Could you check a few things on this model? Use its own coordinates, in mm. Round coordinates to 2 decimals unless told otherwise and drop trailing zeros. Loops run counter-clockwise (first coordinate to the right, second up) from the corner with the lowest first, then second, coordinate; pieces in that order, holes last. Notation, with made-up numbers: (41, 27) - (57, 27) arc R31 cw to (57, 56) - close; hole circle Ø2 at (-15, 88.5). An arc over 180 degrees is marked (long way). Use one line per item in the form item = value.
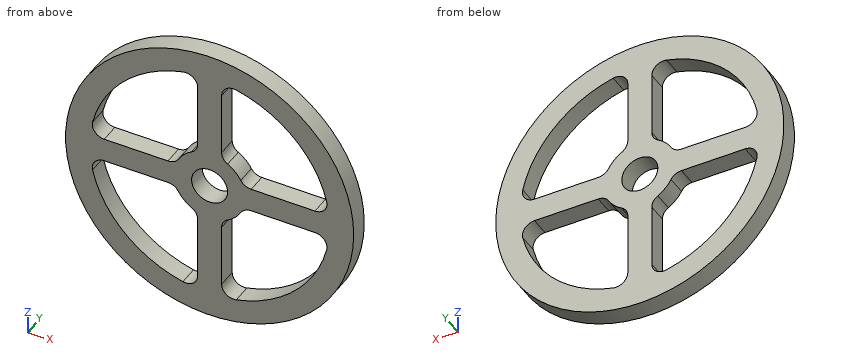
```python
from build123d import *

# Parameters (mm, degrees)
SKETCH1_R           = 120
SKETCH1_R_2         = 15
BOSS_EXTRUDE1_DEPTH = 16


with BuildPart() as part:
    # Sketch1 → Boss-Extrude1 (new body)
    with BuildSketch(Plane(origin=(0, 0, 0), x_dir=(1, 0, 0), z_dir=(0, 1, 0))):
        Circle(SKETCH1_R)
        Circle(SKETCH1_R_2, mode=Mode.SUBTRACT)
        with BuildLine():
            Line((34.641016151, 10), (87.749643874, 10))
            ThreePointArc((87.749643874, 10), (95.567003474, 13.763904355), (97.499604304, 22.222222222))
            ThreePointArc((97.499604304, 22.222222222), (70.710678119, 70.710678119), (22.222222222, 97.499604304))
            ThreePointArc((22.222222222, 97.499604304), (13.763904355, 95.567003474), (10, 87.749643874))
            Line((10, 87.749643874), (10, 34.641016151))
            ThreePointArc((10, 34.641016151), (11.339745962, 29.641016151), (15, 25.980762114))
            ThreePointArc((15, 25.980762114), (21.213203436, 21.213203436), (25.980762114, 15))
            ThreePointArc((25.980762114, 15), (29.641016151, 11.339745962), (34.641016151, 10))
        make_face(mode=Mode.SUBTRACT)
        with BuildLine():
            Line((-10, 34.641016151), (-10, 87.749643874))
            ThreePointArc((-10, 87.749643874), (-13.763904355, 95.567003474), (-22.222222222, 97.499604304))
            ThreePointArc((-22.222222222, 97.499604304), (-70.710678119, 70.710678119), (-97.499604304, 22.222222222))
            ThreePointArc((-97.499604304, 22.222222222), (-95.567003474, 13.763904355), (-87.749643874, 10))
            Line((-87.749643874, 10), (-34.641016151, 10))
            ThreePointArc((-34.641016151, 10), (-29.641016151, 11.339745962), (-25.980762114, 15))
            ThreePointArc((-25.980762114, 15), (-21.213203436, 21.213203436), (-15, 25.980762114))
            ThreePointArc((-15, 25.980762114), (-11.339745962, 29.641016151), (-10, 34.641016151))
        make_face(mode=Mode.SUBTRACT)
        with BuildLine():
            Line((34.641016151, -10), (87.749643874, -10))
            ThreePointArc((87.749643874, -10), (95.567003474, -13.763904355), (97.499604304, -22.222222222))
            ThreePointArc((97.499604304, -22.222222222), (70.710678119, -70.710678119), (22.222222222, -97.499604304))
            ThreePointArc((22.222222222, -97.499604304), (13.763904355, -95.567003474), (10, -87.749643874))
            Line((10, -87.749643874), (10, -34.641016151))
            ThreePointArc((10, -34.641016151), (11.339745962, -29.641016151), (15, -25.980762114))
            ThreePointArc((15, -25.980762114), (21.213203436, -21.213203436), (25.980762114, -15))
            ThreePointArc((25.980762114, -15), (29.641016151, -11.339745962), (34.641016151, -10))
        make_face(mode=Mode.SUBTRACT)
        with BuildLine():
            Line((-10, -34.641016151), (-10, -87.749643874))
            ThreePointArc((-10, -87.749643874), (-13.763904355, -95.567003474), (-22.222222222, -97.499604304))
            ThreePointArc((-22.222222222, -97.499604304), (-70.710678119, -70.710678119), (-97.499604304, -22.222222222))
            ThreePointArc((-97.499604304, -22.222222222), (-95.567003474, -13.763904355), (-87.749643874, -10))
            Line((-87.749643874, -10), (-34.641016151, -10))
            ThreePointArc((-34.641016151, -10), (-29.641016151, -11.339745962), (-25.980762114, -15))
            ThreePointArc((-25.980762114, -15), (-21.213203436, -21.213203436), (-15, -25.980762114))
            ThreePointArc((-15, -25.980762114), (-11.339745962, -29.641016151), (-10, -34.641016151))
        make_face(mode=Mode.SUBTRACT)
    extrude(amount=BOSS_EXTRUDE1_DEPTH)


solid = part.part
```
1. If we section it at A-A, the plane y = 6.25: Count the separate pieces of the cut face and the enclosed holes in it, plus the area to 3 significant figures.
Solution:
separate_pieces = 1
enclosed_holes = 5
area = 21,900 mm^2
2. If we section it at B-B, the plane x = 0: Write out the boundary of the cut face in (y, z).
Solution:
outline = (0, -120) - (16, -120) - (16, -15) - (0, -15) - close; (0, 15) - (16, 15) - (16, 120) - (0, 120) - close
3. If we section it at C-C, the plane z = 0: Write out the boundary of the cut face in (x, y), plus the area to 3 significant figures.
Solution:
outline = (-120, 0) - (-15, 0) - (-15, 16) - (-120, 16) - close; (15, 0) - (120, 0) - (120, 16) - (15, 16) - close
area = 3,360 mm^2
4. For P1, Ø8, axis at x = 71.5, y = 2, coming from the -Z side; P2, Ø8, axis at x = 71.5, y = 8, coming from the +Z side; P3, Ø2, axis at x = -78, y = 8.5, coming from the +Z side; P4, Ø1, axis at y = 12.5, z = 0.5, coming from the +X side, each with a flat end and sliding along its axis, tell me the tip position at first contact or that it passes through.
Solution:
P1 = -99.22
P2 = 99.22
P3 = 92.04
P4 = 120
5. Please list where these lines run through material, in increasing order: line 1 along Z through (x, y) = (0, 8); line 2 along X through (y, z) = (7.75, -16).
Solution:
line_1 = -120 to -15, 15 to 120
line_2 = -118.93 to -96.91, -25.38 to 25.38, 96.91 to 118.93
6. If we section it at D-D, the plane x = 53: Write out the boundary of the cut face in (y, z), plus the area to 3 significant figures.
Solution:
outline = (0, -107.66) - (16, -107.66) - (16, -84.8) - (0, -84.8) - close; (0, -10) - (16, -10) - (16, 10) - (0, 10) - close; (0, 84.8) - (16, 84.8) - (16, 107.66) - (0, 107.66) - close
area = 1,050 mm^2
